Input: dimensioned drawing with shaded views. Units: mm. Origin: part minimum x, y, z. Round coordinates to 2 decimals unless told otherwise and drop trailing zeros. Loops run counter-clockwise (first coordinate to the right, second up) from the corner with the lowest first, then second, coordinate; pieces in that order, holes last.
1) Section B-B, the plane z = 1.1. State how many separate pieces and enclosed holes the cut face has, and give its area (3 significant figures).
2) Section C-C, the plane y = 74. Return loops of the section in (x, z).
3) Ray query, line 1 along Y through (x, z) = (137, 1.05); line 2 along X through (y, z) = (140.5, 1.2); line 3 along Y through (x, z) = (97, 0.7) (3 decimals). Return the intervals inside material, ascending.
4) First-contact query: pin 1 (1.5 mm diameter, centred on y = 149.5, z = 3, fed in from +X); pin 2 (4 mm diameter, centred on x = 63, y = 179.05, fed in from +Z); pin 3 (2 mm diameter, centred on x = 120.5, z = 2.5, fed in from +Y). Flat tips, straight axial feed; report the tip coordinate or a pass-through.
5) Section D-D, the plane x = 27.5. Return loops of the section in (y, z) (3 decimals).
6) Section A-A, the plane x = 63. Return loops of the section in (y, z), and give its area (3 significant figures).
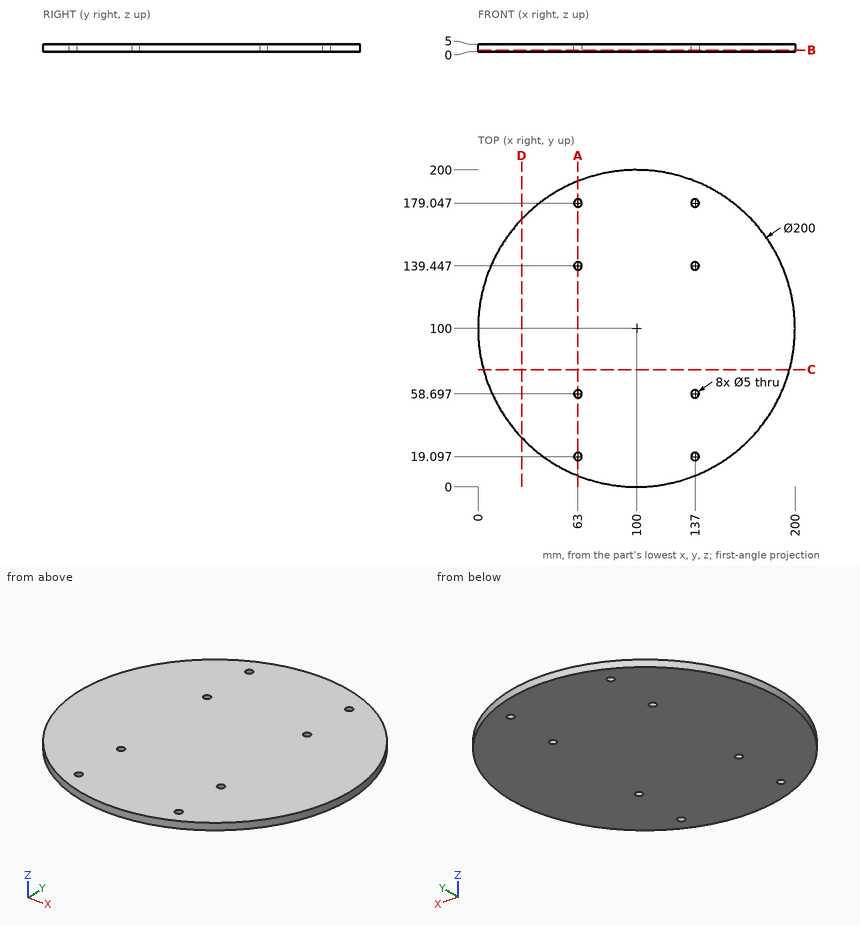
Final values:
1. separate pieces: 1
1. enclosed holes: 8
1. area: 31,300 mm2
2. outline: (3.44, 0) - (196.56, 0) - (196.56, 5) - (3.44, 5) - close
3. line 1: y = 7.1 to 16.6, 21.6 to 56.2, 61.2 to 136.95, 141.95 to 176.55, 181.55 to 192.9
3. line 2: x = 8.57 to 60.73, 65.27 to 134.73, 139.27 to 191.43
3. line 3: y = 0.045 to 199.955
4. pin 1: stops at x = 187.31
4. pin 2: passes through
4. pin 3: stops at y = 198.08
5. outline: (31.125, 0) - (168.875, 0) - (168.875, 5) - (31.125, 5) - close
6. outline: (7.1, 0) - (16.6, 0) - (16.6, 5) - (7.1, 5) - close; (21.6, 0) - (56.2, 0) - (56.2, 5) - (21.6, 5) - close; (61.2, 0) - (136.95, 0) - (136.95, 5) - (61.2, 5) - close; (141.95, 0) - (176.55, 0) - (176.55, 5) - (141.95, 5) - close; (181.55, 0) - (192.9, 0) - (192.9, 5) - (181.55, 5) - close
6. area: 829 mm2
